```python
from build123d import *

# Parameters (mm, degrees)
SKETCH1_W           = 65
SKETCH1_H           = 65
SKETCH1_R           = 3
BOSS_EXTRUDE1_DEPTH = 6
FILLET1_R           = 5
SKETCH2_W           = 41
SKETCH2_H           = 4
BOSS_EXTRUDE2_DEPTH = 8
FILLET2_R           = 2
SKETCH3_R           = 2.5
CUT_EXTRUDE1_DEPTH  = 15
SKETCH_1_R          = 1.75
CUT_EXTRUDE_1_DEPTH = 66


with BuildPart() as part:
    # Sketch1 → Boss-Extrude1 (new body)
    with BuildSketch(Plane.XY):
        Rectangle(SKETCH1_W, SKETCH1_H)
        with Locations((25, 26.5)):
            Circle(SKETCH1_R, mode=Mode.SUBTRACT)
        with Locations((25, -23.5)):
            Circle(SKETCH1_R, mode=Mode.SUBTRACT)
        with Locations((-25, -23.5)):
            Circle(SKETCH1_R, mode=Mode.SUBTRACT)
        with Locations((-25, 26.5)):
            Circle(SKETCH1_R, mode=Mode.SUBTRACT)
    extrude(amount=BOSS_EXTRUDE1_DEPTH)

    # Fillet1
    fillet1_edges = [part.edges().sort_by_distance(p)[0] for p in [
        (32.5, -32.5, 3),
        (-32.5, -32.5, 3),
        (-32.5, 32.5, 3),
        (32.5, 32.5, 3),
    ]]
    fillet(fillet1_edges, radius=FILLET1_R)

    # Sketch2 → Boss-Extrude2 (add)
    with BuildSketch(Plane.XY.offset(6)):
        with Locations((0, -30.5)):
            Rectangle(SKETCH2_W, SKETCH2_H)
    extrude(amount=BOSS_EXTRUDE2_DEPTH)

    # Fillet2
    fillet2_edges = [part.edges().sort_by_distance(p)[0] for p in [
        (-20.5, -30.5, 6),
        (20.5, -30.5, 6),
        (-20.5, -30.5, 14),
        (20.5, -30.5, 14),
    ]]
    fillet(fillet2_edges, radius=FILLET2_R)

    # Sketch3 → Cut-Extrude1 (cut, through all)
    with BuildSketch(Plane(origin=(0, 0, 0), x_dir=(-1, 0, 0), z_dir=(0, 0, -1))):
        with Locations((-15, 25)):
            Circle(SKETCH3_R)
        with Locations((15, 25)):
            Circle(SKETCH3_R)
        with Locations((-15, -15)):
            Circle(SKETCH3_R)
        with Locations((15, -15)):
            Circle(SKETCH3_R)
    extrude(amount=-CUT_EXTRUDE1_DEPTH, mode=Mode.SUBTRACT)

    # 草图1 → 切除-拉伸1 (cut, through all)
    with BuildSketch(Plane.XZ.offset(32.5)):
        with Locations((-16, 10)):
            Circle(SKETCH_1_R)
        with Locations((0, 10)):
            Circle(SKETCH_1_R)
        with Locations((16, 10)):
            Circle(SKETCH_1_R)
    extrude(amount=-CUT_EXTRUDE_1_DEPTH, mode=Mode.SUBTRACT)


solid = part.part
```
Could you check a few things on this model? Use its own coordinates, in mm. A direction names the side the tool comes from. Give positions to 0.01 mm unless a question says otherwise; leave off trailing zeros. Write each loop counter-clockwise with the first axis right and the second up, starting at its lowest first coordinate (ties: lowest second). Pieces come first, ordered by that corner, then holes. Notation, with made-up numbers: (-14, 40.5) -> (3, 40.5) arc R9 ccw to (3, 54.5) -> close; hole circle Ø5 at (53.25, -26). An arc over 180 degrees is marked (long way). Write each question's results on one line, items separated by ' | '.
1. I want a section at B-B, the plane z = 10. Write out the boundary of the cut face in (x, y), then the cut area to 3 significant figures.
Check sheet entries:
outline: (-20.5, -32.5) -> (-17.75, -32.5) -> (-17.75, -28.5) -> (-20.5, -28.5) -> close; (-14.25, -32.5) -> (-1.75, -32.5) -> (-1.75, -28.5) -> (-14.25, -28.5) -> close; (1.75, -32.5) -> (14.25, -32.5) -> (14.25, -28.5) -> (1.75, -28.5) -> close; (17.75, -32.5) -> (20.5, -32.5) -> (20.5, -28.5) -> (17.75, -28.5) -> close | area: 122 mm²
2. I need wall thicknesses on L1, parallel to Y at x = -15, z = 2.1; L2, parallel to Z at x = 16, y = -30.25; L3, parallel to X at y = -29, z = 11. Which ranges of each line are inside material? Lowest first, please.
Check sheet entries:
L1: y = -32.5 to -17.5, -12.5 to 22.5, 27.5 to 32.5 | L2: z = 0 to 8.25, 11.75 to 14 | L3: x = -20.5 to -17.44, -14.56 to -1.44, 1.44 to 14.56, 17.44 to 20.5
3. I want a section at A-A, the plane x = -25. Write out the boundary of the cut face in (y, z), then the cut area to 3 significant figures.
Check sheet entries:
outline: (-32.5, 0) -> (-26.5, 0) -> (-26.5, 6) -> (-32.5, 6) -> close; (-20.5, 0) -> (23.5, 0) -> (23.5, 6) -> (-20.5, 6) -> close; (29.5, 0) -> (32.5, 0) -> (32.5, 6) -> (29.5, 6) -> close | area: 318 mm²
4. I want a section at C-C, the plane y = -15. Write out the boundary of the cut face in (x, z).
Check sheet entries:
outline: (-32.5, 0) -> (-17.5, 0) -> (-17.5, 6) -> (-32.5, 6) -> close; (-12.5, 0) -> (12.5, 0) -> (12.5, 6) -> (-12.5, 6) -> close; (17.5, 0) -> (32.5, 0) -> (32.5, 6) -> (17.5, 6) -> close
5. Will these pins go through, and if not, where does the flat tip stop? pin 1 Ø4.5 at (x, z) = (-16, 10) entering from +Y; pin 2 Ø9.5 at (x, y) = (25, 26.5) entering from +Z; pin 3 Ø1.2 at (y, z) = (-30.5, 10.5) entering from -X.
Check sheet entries:
pin 1: stops at y = -28.5 | pin 2: stops at z = 6 | pin 3: stops at x = -20.5
6. If we mould it in two halves opening along Z, with no side actions, what happens to faces 4 (the cylindrical face through (-0.228, -30.528, 11.735)), 5 (the cylindrical face through (24.35, -26.43, 2.96)), 6 (the flat face through (0, 0, 6))? For each: released by +Z, released by -Z, zero draft, split by the parting line, or undercut.
Check sheet entries:
face 4: undercut | face 5: zero draft | face 6: released by +Z
7. I want a section at D-D, the plane x = -15. Write out the boundary of the cut face in (y, z), then the cut area to 3 significant figures.
Check sheet entries:
outline: (-32.5, 0) -> (-17.5, 0) -> (-17.5, 6) -> (-28.5, 6) -> (-28.5, 8.56) -> (-32.5, 8.56) -> close; (-32.5, 11.44) -> (-28.5, 11.44) -> (-28.5, 14) -> (-32.5, 14) -> close; (-12.5, 0) -> (22.5, 0) -> (22.5, 6) -> (-12.5, 6) -> close; (27.5, 0) -> (32.5, 0) -> (32.5, 6) -> (27.5, 6) -> close | area: 351 mm²
8. On a 3-axis mill with a long thin cutter (end or side, diameter ignored), from which of +Z, -Z, +X, -X, +Y, -Y can I reach the whole of each face in a straight line? I mean faces 1 (the cylindrical face through (17, -16.5, 3)), 2 (the flat face through (-20.5, -31, 10)), 3 (the flat face through (20.5, -31, 10)). Say none if no direction works.
Check sheet entries:
face 1: +Z, -Z | face 2: +Z, -X, +Y, -Y | face 3: +Z, +X, +Y, -Y
